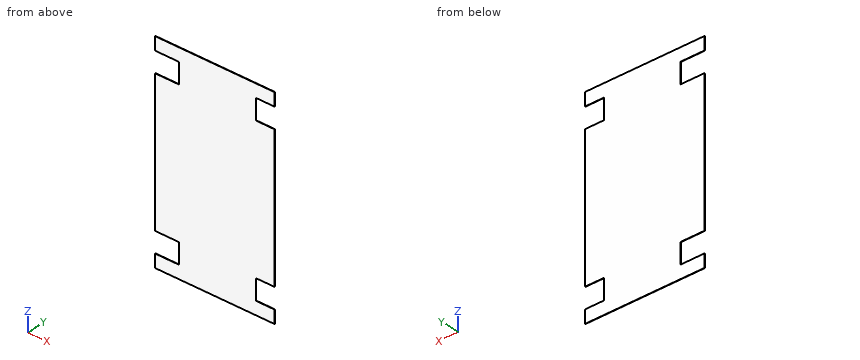
from build123d import *

# Parameters (mm, degrees)
SKETCH1_W           = 469.9
SKETCH1_H           = 812.8
BOSS_EXTRUDE1_DEPTH = 1.5875
SKETCH2_OUTSIDE_W   = 659.672
SKETCH2_OUTSIDE_H   = 1002.572
CUT_EXTRUDE1_DEPTH  = 1.5875


with BuildPart() as part:
    # Sketch1 → Boss-Extrude1 (new body)
    with BuildSketch(Plane(origin=(0, 0, 0), x_dir=(1, 0, 0), z_dir=(0, 1, 0))):
        Rectangle(SKETCH1_W, SKETCH1_H)
    extrude(amount=BOSS_EXTRUDE1_DEPTH)

    # Sketch2 outside → Cut-Extrude1 (cut)
    with BuildSketch(Plane(origin=(0, 1.5875, 0), x_dir=(1, 0, 0), z_dir=(0, 1, 0))):
        Rectangle(SKETCH2_OUTSIDE_W, SKETCH2_OUTSIDE_H)
        Polygon((-234.95, 355.6), (-234.95, 406.4), (234.95, 406.4), (234.95, 355.6), (161.769664855, 355.6), (161.769664855, 276.225), (234.95, 276.225), (234.95, -276.225), (161.769664855, -276.225), (161.769664855, -355.6), (234.95, -355.6), (234.95, -406.4), (-234.95, -406.4), (-234.95, -355.6), (-141.220731077, -355.6), (-141.220731077, -276.225), (-234.95, -276.225), (-234.95, 276.225), (-141.220731077, 276.225), (-141.220731077, 355.6), align=None, mode=Mode.SUBTRACT)
    extrude(amount=-CUT_EXTRUDE1_DEPTH, mode=Mode.SUBTRACT)


solid = part.part
Geometry: final body of the model. Coordinates: model frame, mm. Give positions to 0.01 mm unless a question says otherwise; leave off trailing zeros. Write each loop counter-clockwise with the first axis right and the second up, starting at its lowest first coordinate (ties: lowest second). Pieces come first, ordered by that corner, then holes. Notation, with made-up numbers: (4.25, 59) -> (56.25, 59) arc R31 ccw to (56.25, 90) -> close; hole circle Ø9 at (-2, 6.25). An arc over 180 degrees is marked (long way). Answer as a JSON object with one key per item and string values.
1. Cut plane B-B on y = 1. Output: boundary loops of the cut face in (x, z) (3 decimals), and give its area (3 significant figures).
Ans:
{"outline": "(-234.95, -406.4) -> (234.95, -406.4) -> (234.95, -355.6) -> (161.77, -355.6) -> (161.77, -276.225) -> (234.95, -276.225) -> (234.95, 276.225) -> (161.77, 276.225) -> (161.77, 355.6) -> (234.95, 355.6) -> (234.95, 406.4) -> (-234.95, 406.4) -> (-234.95, 355.6) -> (-141.221, 355.6) -> (-141.221, 276.225) -> (-234.95, 276.225) -> (-234.95, -276.225) -> (-141.221, -276.225) -> (-141.221, -355.6) -> (-234.95, -355.6) -> close", "area": "355,000 mm^2"}
2. Cut plane A-A on x = 187. Output: boundary loops of the cut face in (y, z) (1 decimal).
Ans:
{"outline": "(0, -406.4) -> (1.6, -406.4) -> (1.6, -355.6) -> (0, -355.6) -> close; (0, -276.2) -> (1.6, -276.2) -> (1.6, 276.2) -> (0, 276.2) -> close; (0, 355.6) -> (1.6, 355.6) -> (1.6, 406.4) -> (0, 406.4) -> close"}
3. Ray query, probe 1 along Z at (x, y) = (174, 0.65) (3 decimals); probe 2 along X at (y, z) = (1.2, -302.5). Return the intervals inside material, ascending. Write a range as from..to.
Ans:
{"probe 1": "z = -406.4..-355.6, -276.225..276.225, 355.6..406.4", "probe 2": "x = -141.22..161.77"}
4. Cut plane C-C on z = 308. Output: boundary loops of the cut face in (x, y), and give its area (3 significant figures).
Ans:
{"outline": "(-141.22, 0) -> (161.77, 0) -> (161.77, 1.59) -> (-141.22, 1.59) -> close", "area": "481 mm^2"}
5. Contact query for flat-ended pins moving along their axis: pin 1 (0.8 mm diameter, centred on y = 0.5, z = -335.5, fed in from +X); pin 2 (2 mm diameter, centred on x = -83, z = -107.5, fed in from -Y). Output: stop coordinate, or through.
Ans:
{"pin 1": "stops at x = 161.77", "pin 2": "stops at y = 0"}
